Model file for the job. Use its own axes, mm. Coordinates: 2 decimals unless noted, no trailing zeros. Loops run counter-clockwise (first coordinate to the right, second up) from the corner with the lowest first, then second, coordinate; pieces in that order, holes last.
from build123d import *

# Parameters (mm, degrees)
SKETCH1_R           = 1.75
BOSS_EXTRUDE1_DEPTH = 3


with BuildPart() as part:
    # Sketch1 → Boss-Extrude1 (new body)
    with BuildSketch(Plane.XY):
        with BuildLine():
            Line((10, 0), (90, 0))
            ThreePointArc((90, 0), (97.071067812, 2.928932188), (100, 10))
            Line((100, 10), (100, 65))
            ThreePointArc((100, 65), (97.071067812, 72.071067812), (90, 75))
            Line((90, 75), (10, 75))
            ThreePointArc((10, 75), (2.928932188, 72.071067812), (0, 65))
            Line((0, 65), (0, 10))
            ThreePointArc((0, 10), (2.928932188, 2.928932188), (10, 0))
        make_face()
        with Locations((10, 70.5)):
            Circle(SKETCH1_R, mode=Mode.SUBTRACT)
        with Locations((10, 65.5)):
            Circle(SKETCH1_R, mode=Mode.SUBTRACT)
        with Locations((10, 60.5)):
            Circle(SKETCH1_R, mode=Mode.SUBTRACT)
        with Locations((10, 55.5)):
            Circle(SKETCH1_R, mode=Mode.SUBTRACT)
        with Locations((15, 70.5)):
            Circle(SKETCH1_R, mode=Mode.SUBTRACT)
        with Locations((15, 65.5)):
            Circle(SKETCH1_R, mode=Mode.SUBTRACT)
        with Locations((15, 60.5)):
            Circle(SKETCH1_R, mode=Mode.SUBTRACT)
        with Locations((15, 55.5)):
            Circle(SKETCH1_R, mode=Mode.SUBTRACT)
        with Locations((20, 70.5)):
            Circle(SKETCH1_R, mode=Mode.SUBTRACT)
        with Locations((20, 65.5)):
            Circle(SKETCH1_R, mode=Mode.SUBTRACT)
        with Locations((20, 60.5)):
            Circle(SKETCH1_R, mode=Mode.SUBTRACT)
        with Locations((20, 55.5)):
            Circle(SKETCH1_R, mode=Mode.SUBTRACT)
        with Locations((34.45, 70.5)):
            Circle(SKETCH1_R, mode=Mode.SUBTRACT)
        with Locations((39.45, 70.5)):
            Circle(SKETCH1_R, mode=Mode.SUBTRACT)
        with Locations((44.45, 70.5)):
            Circle(SKETCH1_R, mode=Mode.SUBTRACT)
        with Locations((44.45, 65.5)):
            Circle(SKETCH1_R, mode=Mode.SUBTRACT)
        with Locations((39.45, 65.5)):
            Circle(SKETCH1_R, mode=Mode.SUBTRACT)
        with Locations((34.45, 65.5)):
            Circle(SKETCH1_R, mode=Mode.SUBTRACT)
        with Locations((34.45, 60.5)):
            Circle(SKETCH1_R, mode=Mode.SUBTRACT)
        with Locations((39.45, 60.5)):
            Circle(SKETCH1_R, mode=Mode.SUBTRACT)
        with Locations((44.45, 60.5)):
            Circle(SKETCH1_R, mode=Mode.SUBTRACT)
        with Locations((44.45, 55.5)):
            Circle(SKETCH1_R, mode=Mode.SUBTRACT)
        with Locations((39.45, 55.5)):
            Circle(SKETCH1_R, mode=Mode.SUBTRACT)
        with Locations((34.45, 55.5)):
            Circle(SKETCH1_R, mode=Mode.SUBTRACT)
    extrude(amount=BOSS_EXTRUDE1_DEPTH)


solid = part.part
Q1. Slice it at B-B (x = 34.45). List the corners of the cut face in (y, z).
Answers:
outline: (0, 0) - (53.75, 0) - (53.75, 3) - (0, 3) - close; (57.25, 0) - (58.75, 0) - (58.75, 3) - (57.25, 3) - close; (62.25, 0) - (63.75, 0) - (63.75, 3) - (62.25, 3) - close; (67.25, 0) - (68.75, 0) - (68.75, 3) - (67.25, 3) - close; (72.25, 0) - (75, 0) - (75, 3) - (72.25, 3) - close
Q2. Drill centre lines: line 1 (Y direction, x = 10, z = 0.6); line 2 (Y direction, x = 43.5, z = 0.2); line 3 (X direction, y = 4.5, z = 0.9). Where is each one in solid material? Low to high.
Answers:
line 1: y = 0 to 53.75, 57.25 to 58.75, 62.25 to 63.75, 67.25 to 68.75, 72.25 to 75
line 2: y = 0 to 54.03, 56.97 to 59.03, 61.97 to 64.03, 66.97 to 69.03, 71.97 to 75
line 3: x = 1.65 to 98.35
Q3. Mould opens along Y. For faces 1 (the cylindrical face through (14.62, 58.79, 1.48)), 2 (the flat face through (49, 38, 3)), 3 (the flat face through (51, 75, 1)), 4 (the cylindrical face through (96.99, 2.85, 1.48)) say: +Y half, -Y half, draft (parallel to the pull), parting line (faces both ways), or undercut.
Answers:
face 1: undercut
face 2: draft
face 3: +Y half
face 4: -Y half
Q4. Slice it at C-C (y = 70.5). List the corners of the cut face in (x, z).
Answers:
outline: (1.65, 0) - (8.25, 0) - (8.25, 3) - (1.65, 3) - close; (11.75, 0) - (13.25, 0) - (13.25, 3) - (11.75, 3) - close; (16.75, 0) - (18.25, 0) - (18.25, 3) - (16.75, 3) - close; (21.75, 0) - (32.7, 0) - (32.7, 3) - (21.75, 3) - close; (36.2, 0) - (37.7, 0) - (37.7, 3) - (36.2, 3) - close; (41.2, 0) - (42.7, 0) - (42.7, 3) - (41.2, 3) - close; (46.2, 0) - (98.35, 0) - (98.35, 3) - (46.2, 3) - close
Q5. Slice it at A-A (z = 1.75). Count the separate pieces of the cut face and the enclosed holes in it, and give its area (3 significant figures).
Answers:
separate pieces: 1
enclosed holes: 24
area: 7,180 mm2
